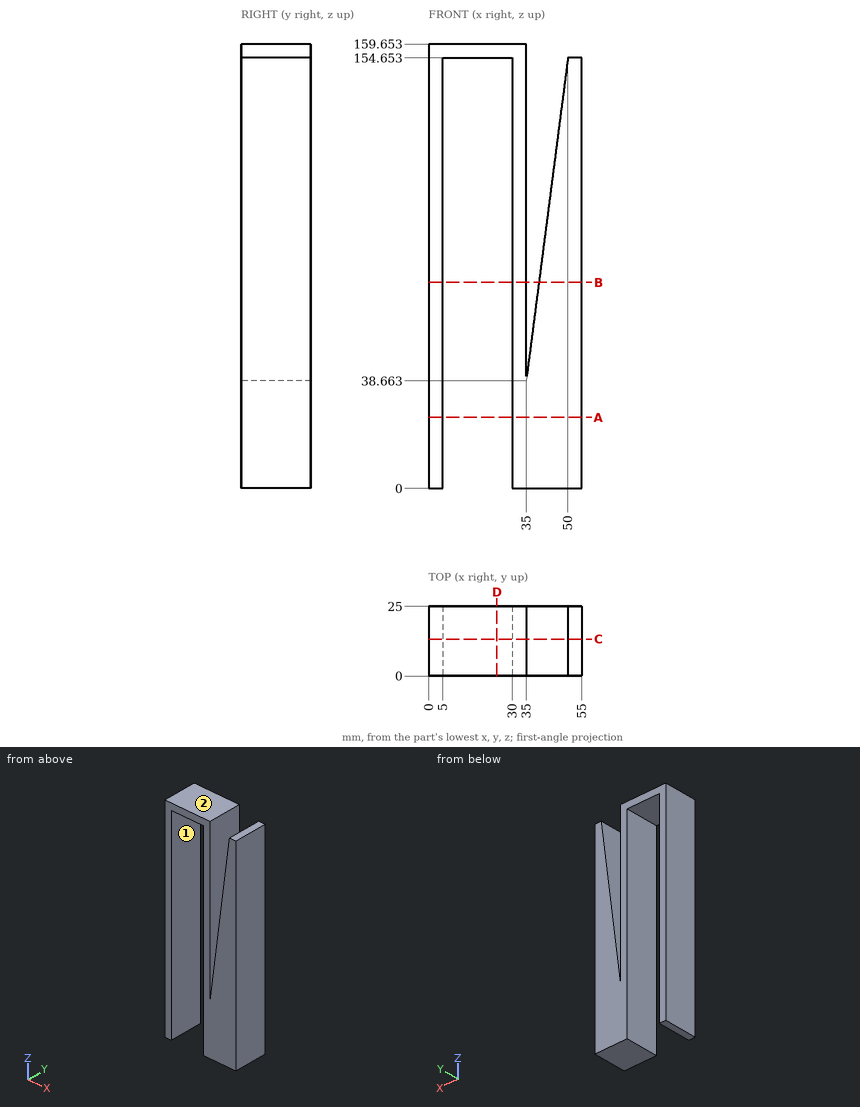
Check sheet for the drawn part. Datum: minimum x, y, z corner. Units: mm. A direction names the side the tool comes from. Round coordinates to 2 decimals unless told otherwise and drop trailing zeros. Write each loop counter-clockwise with the first axis right and the second up, starting at its lowest first coordinate (ties: lowest second). Pieces come first, ordered by that corner, then holes. Notation, with made-up numbers: (9.25, 34.25) -> (26.25, 34.25) arc R19 ccw to (26.25, 60.25) -> close; hole circle Ø10 at (-13.75, 3). An arc over 180 degrees is marked (long way). One line per item, written item: value. Start each with the question number.
(1) Cross-section at A-A, the plane z = 25.5. Record the cut outline in (x, y), and give its area (3 significant figures).
(2) Cross-section at B-B, the plane z = 74. Record the cut outline in (x, y), and give its area (3 significant figures).
(3) Cross-section at D-D, the plane x = 24.5. Record the cut outline in (y, z).
(4) Scan lines: line 1 (X direction, y = 2.5, z = 108); line 2 (X direction, y = 19.25, z = 25); line 3 (X direction, y = 1.75, z = 139.5). Record each from-to range of solid material in increasing order. Write a range as [from, to].
(5) Go/stop test with flat-tipped pins: pin 1 Ø3 at (x, z) = (8, 108) entering from +Y; pin 2 Ø12.5 at (x, y) = (17.5, 17.5) entering from -Z; pin 3 Ø1.5 at (x, y) = (53.5, 9) entering from +Z. Record where each tip stops, or that it passes through.
(6) Cross-section at C-C, the plane y = 13.25. Record the cut outline in (x, z).
(7) Access from +Z, -Z, +X, -X, +Y, -Y to the whole of each face (thin tool, end or side, straight path). Record for the marked faces 1 and 2.
Answer:
1. outline: (0, 0) -> (5, 0) -> (5, 25) -> (0, 25) -> close; (30, 0) -> (55, 0) -> (55, 25) -> (30, 25) -> close
1. area: 750 mm²
2. outline: (0, 0) -> (5, 0) -> (5, 25) -> (0, 25) -> close; (30, 0) -> (35, 0) -> (35, 25) -> (30, 25) -> close; (39.57, 0) -> (55, 0) -> (55, 25) -> (39.57, 25) -> close
2. area: 636 mm²
3. outline: (0, 154.65) -> (25, 154.65) -> (25, 159.65) -> (0, 159.65) -> close
4. line 1: [0, 5], [30, 35], [43.97, 55]
4. line 2: [0, 5], [30, 55]
4. line 3: [0, 5], [30, 35], [48.04, 55]
5. pin 1: through
5. pin 2: z = 154.65
5. pin 3: z = 154.65
6. outline: (0, 0) -> (5, 0) -> (5, 154.65) -> (30, 154.65) -> (30, 0) -> (55, 0) -> (55, 154.65) -> (50, 154.65) -> (35, 38.66) -> (35, 159.65) -> (0, 159.65) -> close
7. face 1: -Z, +Y, -Y
7. face 2: +Z, +X, -X, +Y, -Y
